from build123d import *

# Parameters (mm, degrees)
SKETCH1_R           = 39.6621
BOSS_EXTRUDE2_DEPTH = 7.06
SKETCH5_R           = 1.7653
SKETCH7_R           = 1.575
CUT_EXTRUDE1_DEPTH  = 7.06
BOSS_EXTRUDE4_DEPTH = 7.06
CUT_EXTRUDE2_DEPTH  = 7.06
CHAMFER9_SIZE       = 2.5
CHAMFER10_SIZE      = 2.5
CHAMFER11_SIZE      = 2.5
CHAMFER12_SIZE      = 2.5


with BuildPart() as part:
    # Sketch1 → Boss-Extrude2 (new body)
    with BuildSketch(Plane(origin=(0, 0, 0), x_dir=(1, 0, 0), z_dir=(0, 1, 0))):
        with Locations(Location((0, 0, 0), (0, 0, 270))):
            Circle(SKETCH1_R)
    extrude(amount=BOSS_EXTRUDE2_DEPTH)

    # Sketch5 → Cut-Revolve1 (revolve, cut)
    with BuildSketch(Plane(origin=(0, 0, 0), x_dir=(0, 0, -1), z_dir=(1, 0, 0)), mode=Mode.PRIVATE) as cut_revolve1_sk:
        with Locations((39.6621, 3.53)):
            Circle(SKETCH5_R)
    revolve(cut_revolve1_sk.sketch.rotate(Axis((0, 3.53, 0), (0, 1, 0)), 180), axis=Axis((0, 3.53, 0), (0, 1, 0)), mode=Mode.SUBTRACT)

    # Sketch7 → Cut-Extrude1 (cut)
    with BuildSketch(Plane.XZ):
        with Locations(Location((0, 0, 0), (0, 0, 270))):
            Circle(SKETCH7_R)
    extrude(amount=-CUT_EXTRUDE1_DEPTH, mode=Mode.SUBTRACT)

    # Sketch8 → Boss-Extrude4 (add)
    with BuildSketch(Plane.XZ):
        with BuildLine():
            Line((1.173935688, -1.05), (-1.173935688, -1.05))
            ThreePointArc((-1.173935688, -1.05), (0, -1.575), (1.173935688, -1.05))
        make_face()
    extrude(amount=-BOSS_EXTRUDE4_DEPTH)

    # Sketch9 → Cut-Extrude2 (cut)
    with BuildSketch(Plane(origin=(0, 7.06, 0), x_dir=(1, 0, 0), z_dir=(0, 1, 0))):
        with BuildLine():
            Line((-26.778976355, 22.536335668), (-8.866689125, 4.624048438))
            ThreePointArc((-8.866689125, 4.624048438), (-9.238795325, 3.826834324), (-9.539392014, 3))
            Line((-9.539392014, 3), (-34.871191548, 3))
            ThreePointArc((-34.871191548, 3), (-32.335783638, 13.393920133), (-26.778976355, 22.536335668))
        make_face()
        with BuildLine():
            Line((-34.871191548, -3), (-9.539392014, -3))
            ThreePointArc((-9.539392014, -3), (-9.238795325, -3.826834324), (-8.866689125, -4.624048438))
            Line((-8.866689125, -4.624048438), (-26.778976355, -22.536335668))
            ThreePointArc((-26.778976355, -22.536335668), (-32.335783638, -13.393920133), (-34.871191548, -3))
        make_face()
        with BuildLine():
            Line((-22.536335668, -26.778976355), (-4.624048438, -8.866689125))
            ThreePointArc((-4.624048438, -8.866689125), (-3.826834324, -9.238795325), (-3, -9.539392014))
            Line((-3, -9.539392014), (-3, -34.871191548))
            ThreePointArc((-3, -34.871191548), (-13.393920133, -32.335783638), (-22.536335668, -26.778976355))
        make_face()
        with BuildLine():
            Line((3, -9.539392014), (3, -34.871191548))
            ThreePointArc((3, -34.871191548), (13.393920133, -32.335783638), (22.536335668, -26.778976355))
            Line((22.536335668, -26.778976355), (4.624048438, -8.866689125))
            ThreePointArc((4.624048438, -8.866689125), (3.826834324, -9.238795325), (3, -9.539392014))
        make_face()
        with BuildLine():
            Line((8.866689125, -4.624048438), (26.778976355, -22.536335668))
            ThreePointArc((26.778976355, -22.536335668), (32.335783638, -13.393920133), (34.871191548, -3))
            Line((34.871191548, -3), (9.539392014, -3))
            ThreePointArc((9.539392014, -3), (9.238795325, -3.826834324), (8.866689125, -4.624048438))
        make_face()
        with BuildLine():
            Line((9.539392014, 3), (34.871191548, 3))
            ThreePointArc((34.871191548, 3), (32.335783638, 13.393920133), (26.778976355, 22.536335668))
            Line((26.778976355, 22.536335668), (8.866689125, 4.624048438))
            ThreePointArc((8.866689125, 4.624048438), (9.238795325, 3.826834324), (9.539392014, 3))
        make_face()
        with BuildLine():
            Line((3, 34.871191548), (3, 9.539392014))
            ThreePointArc((3, 9.539392014), (3.826834324, 9.238795325), (4.624048438, 8.866689125))
            Line((4.624048438, 8.866689125), (22.536335668, 26.778976355))
            ThreePointArc((22.536335668, 26.778976355), (13.393920133, 32.335783638), (3, 34.871191548))
        make_face()
        with BuildLine():
            Line((-22.536335668, 26.778976355), (-4.624048438, 8.866689125))
            ThreePointArc((-4.624048438, 8.866689125), (-3.826834324, 9.238795325), (-3, 9.539392014))
            Line((-3, 9.539392014), (-3, 34.871191548))
            ThreePointArc((-3, 34.871191548), (-13.393920133, 32.335783638), (-22.536335668, 26.778976355))
        make_face()
    extrude(amount=-CUT_EXTRUDE2_DEPTH, mode=Mode.SUBTRACT)

    # Chamfer9
    chamfer9_edges = [part.edges().sort_by_distance(p)[0] for p in [
        (-13.580192053, 7.06, -17.82283274),
        (-17.82283274, 7.06, -13.580192053),
    ]]
    chamfer(chamfer9_edges, length=CHAMFER9_SIZE)

    # Chamfer10
    chamfer10_edges = [part.edges().sort_by_distance(p)[0] for p in [
        (-13.580192053, 0, -17.82283274),
        (-17.82283274, 0, -13.580192053),
    ]]
    chamfer(chamfer10_edges, length=CHAMFER10_SIZE)

    # Chamfer11
    chamfer11_edges = [part.edges().sort_by_distance(p)[0] for p in [
        (-9.238795325, 7.06, 3.826834324),
        (-22.205291781, 7.06, 3),
        (-32.335783638, 7.06, 13.393920133),
        (-17.82283274, 7.06, 13.580192053),
        (-3.826834324, 7.06, 9.238795325),
        (-13.580192053, 7.06, 17.82283274),
        (-13.393920133, 7.06, 32.335783638),
        (-3, 7.06, 22.205291781),
        (13.393920133, 7.06, 32.335783638),
        (3, 7.06, 22.205291781),
        (3.826834324, 7.06, 9.238795325),
        (13.580192053, 7.06, 17.82283274),
        (9.238795325, 7.06, 3.826834324),
        (17.82283274, 7.06, 13.580192053),
        (32.335783638, 7.06, 13.393920133),
        (22.205291781, 7.06, 3),
        (32.335783638, 7.06, -13.393920133),
        (22.205291781, 7.06, -3),
        (17.82283274, 7.06, -13.580192053),
        (9.238795325, 7.06, -3.826834324),
        (3.826834324, 7.06, -9.238795325),
        (13.580192053, 7.06, -17.82283274),
        (13.393920133, 7.06, -32.335783638),
        (3, 7.06, -22.205291781),
        (-14.541651461, 7.06, -31.836148837),
        (-3, 7.06, -22.205291781),
        (-4.969104941, 7.06, -8.678017981),
        (-8.678017981, 7.06, -4.969104941),
        (-22.205291781, 7.06, -3),
        (-31.836148837, 7.06, -14.541651461),
    ]]
    chamfer(chamfer11_edges, length=CHAMFER11_SIZE)

    # Chamfer12
    chamfer12_edges = [part.edges().sort_by_distance(p)[0] for p in [
        (3.826834324, 0, -9.238795325),
        (13.580192053, 0, -17.82283274),
        (13.393920133, 0, -32.335783638),
        (3, 0, -22.205291781),
        (-14.541651461, 0, -31.836148837),
        (-4.969104941, 0, -8.678017981),
        (-3, 0, -22.205291781),
        (-8.678017981, 0, -4.969104941),
        (-31.836148837, 0, -14.541651461),
        (-22.205291781, 0, -3),
        (-17.82283274, 0, 13.580192053),
        (-9.238795325, 0, 3.826834324),
        (-32.335783638, 0, 13.393920133),
        (-22.205291781, 0, 3),
        (-3.826834324, 0, 9.238795325),
        (-13.580192053, 0, 17.82283274),
        (-13.393920133, 0, 32.335783638),
        (-3, 0, 22.205291781),
        (3.826834324, 0, 9.238795325),
        (3, 0, 22.205291781),
        (13.393920133, 0, 32.335783638),
        (13.580192053, 0, 17.82283274),
        (9.238795325, 0, 3.826834324),
        (17.82283274, 0, 13.580192053),
        (32.335783638, 0, 13.393920133),
        (22.205291781, 0, 3),
        (9.238795325, 0, -3.826834324),
        (17.82283274, 0, -13.580192053),
        (22.205291781, 0, -3),
        (32.335783638, 0, -13.393920133),
    ]]
    chamfer(chamfer12_edges, length=CHAMFER12_SIZE)


solid = part.part
CAD build for the part. Positions are in the model's coordinates, mm. A direction names the side the tool comes from. Give positions to 0.01 mm unless a question says otherwise; leave off trailing zeros. Return JSON: item names as keys, results as strings.
Item 1: Tool access for faces 1 (the conical face through (-13.583, 5.515, 33.29)), 2 (the flat face through (3, 4, -22)), 3 (the flat face through (-22.3, 1.3, -1.8)): list every direction of +Z, -Z, +X, -X, +Y, -Y with a clear straight run to the whole face (end or side of a thin tool).
Answer below:
{"face 1": "+Y", "face 2": "+Y, -Y", "face 3": "-Y"}
Item 2: Two-plate mould, pull along X, no slides. Class faces 4 (the flat face through (14.5, 5.79, -17)), 5 (the flat face through (1.7, 1.2, -22.7)): +X half, -X half, draft (parallel to the pull), parting line (faces both ways), or undercut.
Answer below:
{"face 4": "undercut", "face 5": "undercut"}
Item 3: Drill centre lines: probe 1 along Z at (x, y) = (-23.5, 2.25); probe 2 along X at (y, z) = (2.75, -6.5); probe 3 along Z at (x, y) = (-24, 1.25). Where is each one in solid material? Low to high.
Answer below:
{"probe 1": "z = -30.43 to -19.61, -2.75 to 2.75, 19.61 to 30.43", "probe 2": "x = -37.52 to -34.39, -10.74 to 10.74, 34.39 to 37.52", "probe 3": "z = -31.58 to -27.17, -26.47 to -21.53, -1.75 to 1.75, 21.53 to 26.47, 27.17 to 31.58"}
Item 4: Band-saw the part on A-A (x = -30). Give the number of separate pieces and of enclosed holes in the cut face, then the cut area to 3 significant figures.
Answer below:
{"separate pieces": "3", "enclosed holes": "0", "area": "103 mm2"}
Item 5: Drop flat-ended pins along their axis: pin 1 (0.6 mm diameter, centred on x = -18, y = 3, fed in from -Z); pin 2 (2 mm diameter, centred on x = -15.5, y = 5, fed in from -Z); pin 3 (2 mm diameter, centred on y = 0.5, z = -3, fed in from +X); pin 4 (1.9 mm diameter, centred on x = 0, z = 0, fed in from -Y). Give the stop position or say it passes through.
Answer below:
{"pin 1": "stops at z = -33.65", "pin 2": "stops at z = -36.9", "pin 3": "stops at x = 39.61", "pin 4": "passes through"}
